from build123d import *

# Parameters (mm, degrees)
BOSS_EXTRUDE1_DEPTH = 5.334
SKETCH2_W           = 12.7
SKETCH2_H           = 5.334
CUT_EXTRUDE1_DEPTH  = 6.334


with BuildPart() as part:
    # Sketch1 → Boss-Extrude1 (new body)
    with BuildSketch(Plane.XY):
        with BuildLine():
            Line((-38.121026248, 59.736005595), (-38.121026248, 98.090005595))
            Line((-38.121026248, 98.090005595), (12.678973752, 98.090005595))
            Line((12.678973752, 98.090005595), (12.678973752, 59.736005595))
            ThreePointArc((12.678973752, 59.736005595), (-12.721026248, 39.115977854), (-38.121026248, 59.736005595))
        make_face()
    extrude(amount=BOSS_EXTRUDE1_DEPTH)

    # Sketch2 → Cut-Extrude1 (cut, through all)
    with BuildSketch(Plane.XY.offset(5.334)):
        with Locations((-31.771026248, 95.423005595)):
            Rectangle(SKETCH2_W, SKETCH2_H)
        with Locations((6.328973752, 95.423005595)):
            Rectangle(SKETCH2_W, SKETCH2_H)
    extrude(amount=-CUT_EXTRUDE1_DEPTH, mode=Mode.SUBTRACT)


solid = part.part
Verification items for the finished model (mm, model axes). A direction names the side the tool comes from. Give positions to 0.01 mm unless a question says otherwise; leave off trailing zeros. Write each loop counter-clockwise with the first axis right and the second up, starting at its lowest first coordinate (ties: lowest second). Pieces come first, ordered by that corner, then holes. Notation, with made-up numbers: M -14,18.5 L -7,18.5 A17 cw -7,46.5 Z; hole C 1.5,74.25 d10. An arc over 180 degrees is marked long. Put each result on its own line as item: value. Start each with the question number.
1. Go/stop test with flat-tipped pins: pin 1 Ø6 at (x, y) = (4.5, 70) entering from -Z; pin 2 Ø1 at (y, z) = (51, 1) entering from +X; pin 3 Ø2.5 at (y, z) = (95.5, 2) entering from -X. Record where each tip stops, or that it passes through.
2. Draft check along Z on faces 1 (the face through (-12, 69, 0)), 2 (the face through (-12, 69, 5.334)), 3 (the face through (-25.421, 95, 3)). Enter one of: +Z half, -Z half, draft (parallel to the pull), parting line (faces both ways), or undercut.
3. Scan lines: line 1 along Y through (x, z) = (-12, 3.3); line 2 along X through (y, z) = (57, 1.7); line 3 along Y through (x, z) = (-2, 4.85). Record each from-to range of solid material in increasing order. Write a range as [from, to].
4. Section check C-C (y = 57.5). Record the cut outline in (x, z), and give its area (3 significant figures).
5. Set-up check for faces 4 (the face through (-32, 92.756, 3)), 5 (the face through (-0.021, 95, 3)), 6 (the face through (-12.23, 39.12, 2.63)): record each of +Z, -Z, +X, -X, +Y, -Y from which the full face is reachable in a straight line by a thin tool's end or side.
6. Section check A-A (z = 3.65). Record the cut outline in (x, y).
7. Section check B-B (x = -31). Record the cut outline in (y, z), and give its area (3 significant figures).
Answer list:
1. pin 1: z = 0
1. pin 2: x = 9.4
1. pin 3: x = -25.42
2. face 1: -Z half
2. face 2: +Z half
2. face 3: draft
3. line 1: [39.13, 98.09]
3. line 2: [-37.39, 11.95]
3. line 3: [41.43, 98.09]
4. outline: M -37.55,0 L 12.1,0 L 12.1,5.33 L -37.55,5.33 Z
4. area: 265 mm2
5. face 4: +Z, -Z, -X, +Y
5. face 5: +Z, -Z, +X, +Y
5. face 6: +Z, -Z, -Y
6. outline: M -38.12,59.74 A25.95 ccw 12.68,59.74 L 12.68,92.76 L -0.02,92.76 L -0.02,98.09 L -25.42,98.09 L -25.42,92.76 L -38.12,92.76 Z
7. outline: M 46.64,0 L 92.76,0 L 92.76,5.33 L 46.64,5.33 Z
7. area: 246 mm2
